The listing builds one solid part. Answer for the finished solid, in the listing's coordinates (mm). Give positions to 0.01 mm unless a question says otherwise; leave off trailing zeros. Loops run counter-clockwise (first coordinate to the right, second up) from the corner with the lowest first, then second, coordinate; pieces in that order, holes last. Notation, with made-up numbers: (35, -17.75) - (85, -17.75) arc R14 cw to (85, 9.25) - close; hole circle Ø7 at (49, 27). An arc over 180 degrees is marked (long way). Write item = value, one per line. Start each with the question number.
1) The mould has two halves that part along Z. Classify faces 1 (the cylindrical face through (-2.934, -16.576, 54.885)), 2 (the flat face through (-0.1, 15.2, -95)), 3 (the cylindrical face through (-14.985, 0.66, 1.33)): +Z half, -Z half, draft (parallel to the pull), parting line (faces both ways), or undercut.
2) Flat-ended cylindrical pins translate along their axes: P1, Ø4.5, axis at x = 0, z = -54.5, coming from the -Y side; P2, Ø2, axis at x = -9.5, z = -47, coming from the -Y side; P3, Ø6, axis at x = 6, z = 36.5, coming from the -Y side; P4, Ø2, axis at x = -8, z = -38.5, coming from the +Y side. Find the tip coordinate at first contact, or state that the pin passes through.
3) Consider probe 1 along Z at (x, y) = (0, -15.9); probe 2 along Y at (x, z) = (0, 47); probe 3 along X at (y, z) = (13.5, -81.5). Determine where each line is inside the solid, lowest interval first.
4) The part is cut by section A-A on y = 0. Write down the section's boundary in (x, z).
5) The part is cut by section C-C on z = -54.5. Write down the section's boundary in (x, y), plus the area to 3 significant figures.
6) The part is cut by section B-B on x = 0. Write down the section's boundary in (y, z).
Autodesk Inventor part; units mm, degrees
ref_plane "Work Plane4" through (0, 18.5, 0) normal (0, 1, 0) x (-1, 0, 0)
ref_plane "YZ Plane" through (0, 0, 0) normal (1, 0, 0) x (0, 1, 0)
ref_plane "XZ Plane" through (0, 0, 0) normal (0, 1, 0) x (-1, 0, 0)
sketch "Sketch1" plane through (0, 0, 0) normal (0, 0, 1) x (1, 0, 0)
  circle A0 centre (0, 0) radius 18.5
  circle A1 centre (0, 0) radius 15
  dimension "d0" = 37
  dimension "d1" = 30
extrude "Extrusion1" add sketch "Sketch1" along normal mid plane 190
ref_plane "Work Plane4" through (0, 18.5, 0) normal (0, 1, 0) x (-1, 0, 0)
sketch "Sketch4" plane through (0, 18.5, 0) normal (0, 1, 0) x (-1, 0, 0)
  line L0 (-18.5, -95) -> (18.5, -95)
  line L1 (18.5, -95) -> (18.5, 95)
  line L2 (-18.5, -95) -> (18.5, -95)
  line L3 (18.5, 95) -> (-18.5, 95)
  point P0 (0, 0)
  point P1 (0, -54.5)
  dimension "d14" = 40.5
  dimension "d22" = 190
  dimension "d23" = 18.5
hole "Hole1" at (0, 18.5, -54.5) direction (0, -1, 0) diameter 5.9175 depth 19.1 tip angle 118
mirror "Mirror1" about plane through (0, 0, 0) normal (0, 0, 1) of "Hole1"
mirror "Mirror2" about plane through (0, 0, 0) normal (0, 1, 0) of "Hole1", "Mirror1"
properties part number "EjeRodilla" material "PLA"
Answer below:
q1.face_1 = undercut
q1.face_2 = -Z half
q1.face_3 = draft
q2.P1 = through
q2.P2 = -16.43
q2.P3 = -18.26
q2.P4 = 17.12
q3.probe_1 = -95 to -57.46, -51.54 to 51.54, 57.46 to 95
q3.probe_2 = -18.5 to -15, 15 to 18.5
q3.probe_3 = -12.65 to -6.54, 6.54 to 12.65
q4.outline = (-18.5, -95) - (-15, -95) - (-15, 95) - (-18.5, 95) - close; (15, -95) - (18.5, -95) - (18.5, 95) - (15, 95) - close
q5.outline = (-2.96, -18.26) - (-2.96, -14.71) arc R15 cw to (-2.96, 14.71) - (-2.96, 18.26) arc R18.5 ccw to start; (2.96, -18.26) arc R18.5 ccw to (2.96, 18.26) - (2.96, 14.71) arc R15 cw to (2.96, -14.71) - close
q5.area = 327 mm2
q6.outline = (-18.5, -95) - (-15, -95) - (-15, -57.46) - (-18.5, -57.46) - close; (-18.5, -51.54) - (-15, -51.54) - (-15, 51.54) - (-18.5, 51.54) - close; (-18.5, 57.46) - (-15, 57.46) - (-15, 95) - (-18.5, 95) - close; (15, -95) - (18.5, -95) - (18.5, -57.46) - (15, -57.46) - close; (15, -51.54) - (18.5, -51.54) - (18.5, 51.54) - (15, 51.54) - close; (15, 57.46) - (18.5, 57.46) - (18.5, 95) - (15, 95) - close
